Read the model definition and answer for the solid it produces. Units are mm, in the model's axes. A direction names the side the tool comes from. Give positions to 0.01 mm unless a question says otherwise; leave off trailing zeros. Write each loop counter-clockwise with the first axis right and the second up, starting at its lowest first coordinate (ties: lowest second). Pieces come first, ordered by that corner, then holes. Notation, with made-up numbers: M 72.25,84 L 109.25,84 A15 ccw 109.25,99 Z; hole C -20,-22 d8. An arc over 180 degrees is marked long. Put each result on its own line as item: value.
Autodesk Inventor part; units mm, degrees
sketch "Sketch1" plane through (0, 0, 0) normal (0, 1, 0) x (-1, 0, 0)
  line L0 (-10, 10) -> (10, 10)
  line L1 (10, 10) -> (10, -10)
  line L2 (10, -10) -> (-10, -10)
  line L3 (-10, -10) -> (-10, 10)
  line L4 (-10, 10) -> (10, -10) construction
  line L5 (10, 10) -> (-10, -10) construction
  circle A0 centre (0, 0) radius 2.4
  dimension "d0" = 20
  dimension "d3" = 4.8
extrude "Extrusion1" add sketch "Sketch1" along normal mid plane 8 contours A0
extrude "Extrusion2" add sketch "Sketch1" along normal blind 4
fillet "Fillet1" radius 2 4 edges at (-10, 4, 0) (0, 4, -10) (10, 4, 0) (0, 4, 10)
properties part number "tampa_001_001_3DPrint"
(1) Section B-B on x = 0 is taken. Determine the outline of the cut face in (y, z).
Result:
outline: M -4,-2.4 L 0,-2.4 L 0,-10 L 2,-10 A2 ccw 4,-8 L 4,8 A2 ccw 2,10 L 0,10 L 0,2.4 L -4,2.4 Z
(2) Section D-D on x = -7.5 is taken. Determine the outline of the cut face in (y, z), and give its area (3 significant figures).
Result:
outline: M 0,-10 L 2,-10 A2 ccw 4,-8 L 4,8 A2 ccw 2,10 L 0,10 Z
area: 78.3 mm²
(3) Section A-A on z = 0 is taken. Determine the outline of the cut face in (x, y), and give its area (3 significant figures).
Result:
outline: M -10,0 L -2.4,0 L -2.4,-4 L 2.4,-4 L 2.4,0 L 10,0 L 10,2 A2 ccw 8,4 L -8,4 A2 ccw -10,2 Z
area: 97.5 mm²
(4) Straight lines are drawn through the part: line 1 along Y through (x, z) = (-3.25, -6.75); line 2 along Z through (x, y) = (1.25, -0.5); line 3 along Y through (x, z) = (-0.25, -9). For each, find the intervals that lie inside material, in ascending order. Write a range as from..to.
Result:
line 1: y = 0..4
line 2: z = -2.05..2.05
line 3: y = 0..3.73
(5) Given pin 1 Ø4 at (x, y) = (1, -2.5) entering from +Z; pin 2 Ø5 at (x, z) = (1.5, -6) entering from -Y, each flat-ended and moving along its own axis, determine where each tip first touches the part or whether it passes through.
Result:
pin 1: stops at z = 2.4
pin 2: stops at y = 0
(6) Which of the six approach directions +Z, -Z, +X, -X, +Y, -Y give full straight-line access (tool end or side, diameter ignored) to faces 1 (the face through (0, 1, 10)), 2 (the face through (2, 0, -2))?
Result:
face 1: +Z, +X, -X, +Y, -Y
face 2: -Y
(7) Section C-C on y = -3 is taken. Determine the outline of the cut face in (x, z).
Result:
outline: C 0,0 d4.8
